from build123d import *

# Parameters (mm, degrees)
F1_DEPTH = 2
F3_D     = 5


with BuildPart() as f1:
    # F0 (on Top) → F1 (new body)
    with BuildSketch(Plane.XY):
        with BuildLine():
            ThreePointArc((37.5, 7.5), (36.035534, 11.035534), (32.5, 12.5))
            Line((32.5, 12.5), (-32.5, 12.5))
            ThreePointArc((-32.5, 12.5), (-36.035534, 11.035534), (-37.5, 7.5))
            Line((-37.5, 7.5), (-37.5, -7.5))
            ThreePointArc((-37.5, -7.5), (-36.035534, -11.035534), (-32.5, -12.5))
            Line((-32.5, -12.5), (32.5, -12.5))
            ThreePointArc((32.5, -12.5), (36.035534, -11.035534), (37.5, -7.5))
            Line((37.5, -7.5), (37.5, 7.5))
        make_face()
    extrude(amount=F1_DEPTH)

    # F3 (through all)
    with Locations(Plane.XY.offset(2)):
        with Locations((-32.5, 7.5)):
            Hole(F3_D / 2)


solid = f1.part
Verification items for the finished model (mm, model axes). Coordinates: 2 decimals unless noted, no trailing zeros. Order: outer loops, then holes, each group sorted by start corner. A loop starts at its lowest first (then second) coordinate and runs counter-clockwise, first axis right, second up. Notation, with made-up numbers: M 33,87 L 53,87 A20 ccw 53,116 Z; hole C 19,65.25 d7. An arc over 180 degrees is marked long. One line per item, written item: value. Start each with the question number.
Item 1: Gauge pin test, flat ends, axial feed: pin 1 (3 mm diameter, centred on x = -32.5, y = 7.5, fed in from -Z); pin 2 (3 mm diameter, centred on x = 3, y = 4.5, fed in from -Z). Record the tip position at first contact, or that the pin passes through.
Item 2: Scan lines: probe 1 along Y at (x, z) = (-32.5, 0.8); probe 2 along X at (y, z) = (8, 0.3); probe 3 along X at (y, z) = (6.5, 0.75). Record each from-to range of solid material in increasing order.
Item 3: Mould release check, pull along X, two halves, no side actions. Record for faces 1 (the cylindrical face through (-31.96, 5.06, 0.99)), 2 (the cylindrical face through (36.07, 11, 0.99)), 3 (the flat face through (-37.5, 0, 1)): released by +X, released by -X, zero draft, split by the parting line, or undercut.
Item 4: Sectioned sample at B-B (y = 8.25). Enter the section's corners in (x, z), then the cut area to 3 significant figures.
Item 5: Sectioned sample at C-C (y = -10.25). Enter the section's corners in (x, z).
Item 6: Sectioned sample at A-A (z = 0.9). Enter the section's corners in (x, y), then the cut area to 3 significant figures.
Conclusion:
1. pin 1: passes through
1. pin 2: stops at z = 0
2. probe 1: y = -12.5 to 5, 10 to 12.5
2. probe 2: x = -37.47 to -34.95, -30.05 to 37.47
2. probe 3: x = -37.5 to -34.79, -30.21 to 37.5
3. face 1: undercut
3. face 2: released by +X
3. face 3: released by -X
4. outline: M -37.44,0 L -34.88,0 L -34.88,2 L -37.44,2 Z; M -30.12,0 L 37.44,0 L 37.44,2 L -30.12,2 Z
4. area: 140 mm^2
5. outline: M -36.68,0 L 36.68,0 L 36.68,2 L -36.68,2 Z
6. outline: M -37.5,-7.5 A5 ccw -32.5,-12.5 L 32.5,-12.5 A5 ccw 37.5,-7.5 L 37.5,7.5 A5 ccw 32.5,12.5 L -32.5,12.5 A5 ccw -37.5,7.5 Z; hole C -32.5,7.5 d5
6. area: 1,830 mm^2
